Build history of the part. All positions in model axes, mm. A direction names the side the tool comes from. Round coordinates to 2 decimals unless told otherwise and drop trailing zeros. Loops run counter-clockwise (first coordinate to the right, second up) from the corner with the lowest first, then second, coordinate; pieces in that order, holes last. Notation, with made-up numbers: M 85.25,89.5 L 131.25,89.5 A24 ccw 131.25,108.5 Z; hole C 74.25,72.25 d2. An arc over 180 degrees is marked long. Write each question's results on one line, items separated by ' | '. Start each with the question number.
```python
from build123d import *

# Parameters (mm, degrees)
F1_DEPTH = 25.4


# Not quite as in the source:
# - ends of sketch curves that miss each other by under 0.0002 mm in the source are joined


with BuildPart() as f1:
    # F0 (on Front) → F1 (new body)
    with BuildSketch(Plane.XZ):
        Polygon((-2.4299337529, 26.016831398), (-2.4299337529, -46.8811690807), (1.718732994, -46.8811690807), (1.718732994, 26.0008927435), (1.7185925992, 26.0008932828), align=None)
        Polygon((1.718732994, -46.8811690807), (-2.4299337529, -46.8811690807), (0, -50.4371710122), align=None)
        with BuildLine():
            ThreePointArc((-19.7358001024, 35.2624356747), (-9.9254202862, 32.8061351822), (-2.4299337529, 26.016831398))
            Line((-2.4299337529, 26.016831398), (1.7185925992, 26.0008932828))
            ThreePointArc((1.7185925992, 26.0008932828), (9.4088856226, 32.8066016945), (19.3802025169, 35.2624356747))
            Line((19.3802025169, 35.2624356747), (-19.7358001024, 35.2624356747))
        make_face()
    extrude(amount=F1_DEPTH)


solid = f1.part
```
Item 1: Tool access for faces 1 (the flat face through (1.719, -13, -11)), 2 (the flat face through (0, -13, 35.262)), 3 (the flat face through (-2.43, -13, -10)): list every direction of +Z, -Z, +X, -X, +Y, -Y with a clear straight run to the whole face (end or side of a thin tool).
Item 2: Drill centre lines: line 1 along X through (y, z) = (-3.75, 14); line 2 along Z through (x, y) = (-6.5, -18.5); line 3 along Z through (x, y) = (4.5, -1.5). Where is each one in solid material? Low to high. Write a range as [from, to].
Item 3: Saw through at B-B, the plane z = 2.5. Give the cut face in (x, y), then the cut area to 3 significant figures.
Item 4: Drop flat-ended pins along their axis: pin 1 (1.5 mm diameter, centred on y = -17, z = -29.5, fed in from +X); pin 2 (10 mm diameter, centred on y = -5.5, z = 13, fed in from -X). Give the stop position or say it passes through.
Item 5: Saw through at C-C, the plane x = -8.5. Give the cut face in (y, z).
Working result:
1) face 1: -Z, +X, +Y, -Y | face 2: +Z, +X, -X, +Y, -Y | face 3: -Z, -X, +Y, -Y
2) line 1: x = [-2.43, 1.72] | line 2: z = [30.51, 35.26] | line 3: z = [29.27, 35.26]
3) outline: M -2.43,-25.4 L 1.72,-25.4 L 1.72,0 L -2.43,0 Z | area: 105 mm²
4) pin 1: stops at x = 1.72 | pin 2: stops at x = -2.43
5) outline: M -25.4,31.97 L 0,31.97 L 0,35.26 L -25.4,35.26 Z
